Geometry check sheet. Reference: drawing and pictorial views, mm from the part's lowest x, y, z. Round coordinates to 2 decimals unless told otherwise and drop trailing zeros. Order: outer loops, then holes, each group sorted by start corner. A loop starts at its lowest first (then second) coordinate and runs counter-clockwise, first axis right, second up.
(1) Sectioned sample at A-A (y = 15.25). Record the boundary of the cut face in (x, z).
(2) Sectioned sample at C-C (z = 53). Record the boundary of the cut face in (x, y).
(3) Sectioned sample at B-B (x = 9.2). Record the boundary of the cut face in (y, z), plus the area to 3 significant figures.
(4) Sectioned sample at D-D (x = 13.25). Record the boundary of the cut face in (y, z), plus the area to 3 significant figures.
(5) Material ranges on line 1 along Y through (x, z) = (9, 42.5); line 2 along Z through (x, y) = (8.25, 19); line 3 along X through (y, z) = (20.5, 42), recorded low to high.
(6) Go/stop test with flat-tipped pins: pin 1 (4 mm diameter, centred on x = 15, z = 15, fed in from -Y); pin 2 (1 mm diameter, centred on y = 3.5, z = 33.5, fed in from -X); pin 3 (1 mm diameter, centred on x = 13.5, z = 56, fed in from +Y). Record where each tip stops, or that it passes through.
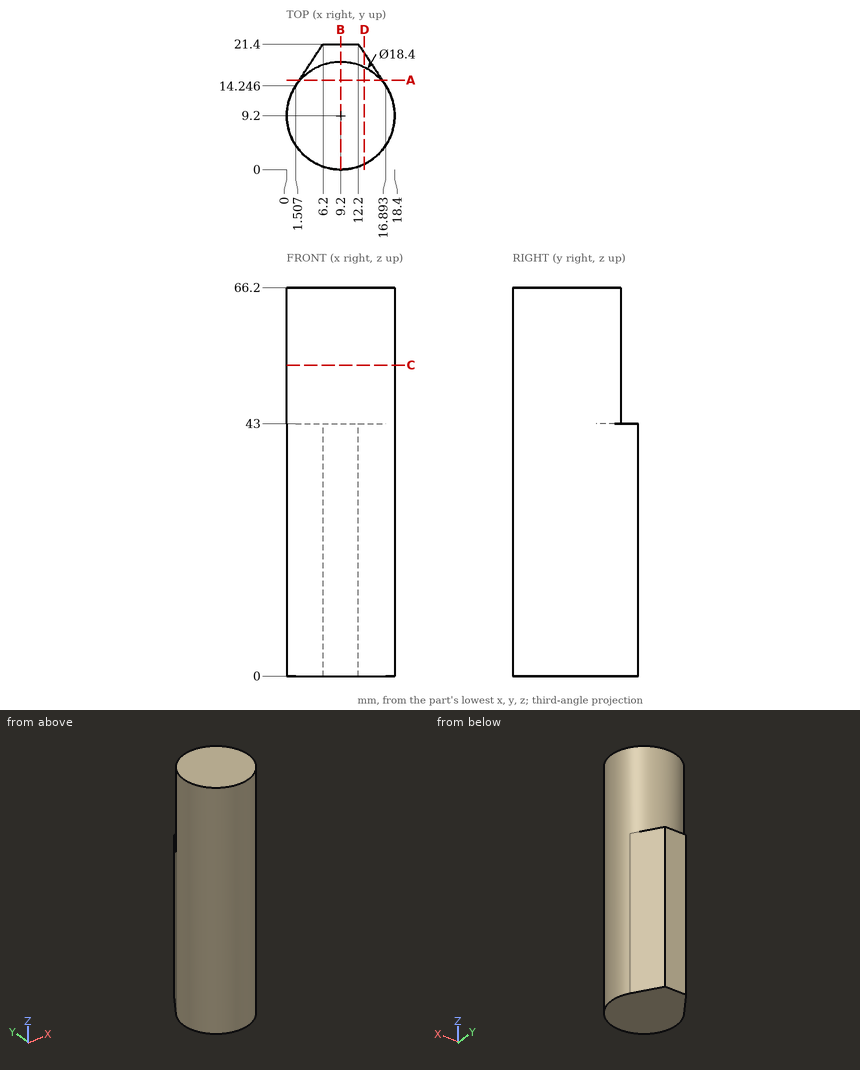
Answer below:
1. outline: (2.17, 0) - (16.23, 0) - (16.23, 43) - (16.13, 43) - (16.13, 66.2) - (2.27, 66.2) - (2.27, 43) - (2.17, 43) - close
2. outline: circle Ø18.4 at (9.2, 9.2)
3. outline: (0, 0) - (21.4, 0) - (21.4, 43) - (18.4, 43) - (18.4, 66.2) - (0, 66.2) - close
3. area: 1,350 mm2
4. outline: (0.94, 0) - (19.8, 0) - (19.8, 43) - (17.46, 43) - (17.46, 66.2) - (0.94, 66.2) - close
4. area: 1,190 mm2
5. line 1: y = 0 to 21.4
5. line 2: z = 0 to 43
5. line 3: x = 5.61 to 12.79
6. pin 1: stops at y = 0.82
6. pin 2: stops at x = 1.61
6. pin 3: stops at y = 17.58
